```python
from build123d import *

# Parameters (mm, degrees)
BASPROSKE_W        = 13
BASPROSKE_H        = 16
TOOTHCUT_DEPTH     = 27.095976701
TEETHCUTS_COUNT    = 14
TEETHCUTS_ANGLE    = 334.285714286
BORSKE_R           = 4
BORE_DEPTH         = 50.0005588
SKETCH2_R          = 0.75
CUT_EXTRUDE1_DEPTH = 6
CIRPATTERN1_COUNT  = 4


with BuildPart() as part:
    # BasProSke → Base-Revolve (revolve)
    with BuildSketch(Plane(origin=(0, 0, 0), x_dir=(1, 0, 0), z_dir=(0, 1, 0)), mode=Mode.PRIVATE) as base_revolve_sk:
        with Locations((6.5, 8)):
            Rectangle(BASPROSKE_W, BASPROSKE_H)
    revolve(base_revolve_sk.sketch.rotate(Axis((-10, 0, 0), (1, 0, 0)), 180), axis=Axis((-10, 0, 0), (1, 0, 0)))

    # TooCutSke → ToothCut (cut, through all)
    with BuildSketch(Plane(origin=(0, 0, 0), x_dir=(0, 0, -1), z_dir=(1, 0, 0))):
        with BuildLine():
            ThreePointArc((1.067858192, 11.449309144), (0, 11.499), (-1.067858192, 11.449309144))
            ThreePointArc((-1.067858192, 11.449309144), (-1.641684211, 13.812780716), (-3.163375005, 15.710076503))
            ThreePointArc((-3.163375005, 15.710076503), (0, 16.0254), (3.163375005, 15.710076503))
            ThreePointArc((3.163375005, 15.710076503), (1.641684211, 13.812780716), (1.067858192, 11.449309144))
        make_face()
    toothcut = extrude(amount=TOOTHCUT_DEPTH, mode=Mode.SUBTRACT)

    # TeethCuts: ToothCut ×14 about axis
    teethcuts_axis = Axis((-10, 0, 0), (1, 0, 0))
    for i in range(1, TEETHCUTS_COUNT):
        add(toothcut.rotate(teethcuts_axis, i * TEETHCUTS_ANGLE / (TEETHCUTS_COUNT - 1)), mode=Mode.SUBTRACT)

    # BorSke → Bore (cut, symmetric)
    with BuildSketch(Plane(origin=(0, 0, 0), x_dir=(0, 0, -1), z_dir=(1, 0, 0))):
        with Locations(Location((0, 0, 0), (0, 0, 180))):
            Circle(BORSKE_R)
    extrude(amount=BORE_DEPTH, both=True, mode=Mode.SUBTRACT)

    # Sketch2 → Cut-Extrude1 (cut)
    with BuildSketch(Plane(origin=(13, 0, 0), x_dir=(0, 0, -1), z_dir=(1, 0, 0))):
        with Locations((-3.5, 7)):
            Circle(SKETCH2_R)
        with Locations((0, 7)):
            Circle(SKETCH2_R)
        with Locations((3.5, 7)):
            Circle(SKETCH2_R)
    cut_extrude1 = extrude(amount=-CUT_EXTRUDE1_DEPTH, mode=Mode.SUBTRACT)

    # CirPattern1: Cut-Extrude1 ×4 about axis
    cirpattern1_axis = Axis((0, 0, 0), (1, 0, 0))
    for i in range(1, CIRPATTERN1_COUNT):
        add(cut_extrude1.rotate(cirpattern1_axis, i * 360 / CIRPATTERN1_COUNT), mode=Mode.SUBTRACT)


solid = part.part
```
Here's how the part is built. I have some questions about the finished solid (model axes, mm). A direction names the side the tool comes from. Round coordinates to 2 decimals unless told otherwise and drop trailing zeros. Order: outer loops, then holes, each group sorted by start corner. A loop starts at its lowest first (then second) coordinate and runs counter-clockwise, first axis right, second up. Notation, with made-up numbers: (73.25, -37) -> (110.25, -37) arc R12 ccw to (110.25, -20) -> close; hole circle Ø1 at (-8.75, 9). An arc over 180 degrees is marked (long way). Use a Markdown table: item, result. Add a question column.
(1) I need wall thicknesses on line 1 along Y through (x, z) = (9.55, -7); line 2 along Z through (x, y) = (7.75, -10); line 3 along Z through (x, y) = (2, -7). Which ranges of each line are inside material? Lowest first, please.
(2) Suppose I cut it at C-C, the plane x = 9.5. Count the separate pieces of the cut face and the enclosed holes in it, and give its area (3 significant figures).
(3) Suppose I cut it at A-A, the plane z = 0. Please give me the cut outline in (x, y), and give its area (3 significant figures).
(4) For faces 4 (the face through (6.409, 10.367, 4.976)), 5 (the face through (10.042, -4.095, 6.544)), 6 (the face through (6.41, -13.77, -1.62)), which set-ups out of +Z, -Z, +X, -X, +Y, -Y let a thin tool reach every point of the face, with its end or its side?
(5) Suppose I cut it at D-D, the plane z = 7. Please give me the cut outline in (x, y).
(6) For pin 1 Ø4 at (x, y) = (11, -9.5) entering from +Z; pin 2 Ø5 at (x, z) = (11, -11) entering from -Y; pin 3 Ø4 at (x, y) = (6, 4.5) entering from +Z; pin 4 Ø5 at (y, z) = (0, 0) entering from -X, each with a flat end and sliding along its axis, tell me the tip position at first contact or that it passes through.
(7) Suppose I cut it at B-B, the plane z = -9. Please give me the cut outline in (x, y), and give its area (3 significant figures).
(8) If we mould it in two halves opening along Z, with no side actions, what happens to faces 1 (the face through (7, 0, -16)), 2 (the face through (6.591, 3.905, -0.867)), 3 (the face through (13, 3, -3))? For each: released by +Z, released by -Z, zero draft, split by the parting line, or undercut.
Verdict:
| question | item | result |
|---|---|---|
| 1 | line 1 | -11.32 to -4.25, -2.75 to -0.75, 0.75 to 2.75, 4.25 to 11.32 |
| 1 | line 2 | -9.82 to -6.01, -5.68 to 5.68, 6.01 to 9.82 |
| 1 | line 3 | -14.39 to -10.8, -9.12 to 9.12, 10.8 to 14.39 |
| 2 | separate pieces | 1 |
| 2 | enclosed holes | 13 |
| 2 | area | 512 mm2 |
| 3 | outline | (0, -11.5) -> (13, -11.5) -> (13, -7.75) -> (7, -7.75) -> (7, -6.25) -> (13, -6.25) -> (13, -4) -> (0, -4) -> close; (0, 4) -> (13, 4) -> (13, 6.25) -> (7, 6.25) -> (7, 7.75) -> (13, 7.75) -> (13, 11.5) -> (0, 11.5) -> close |
| 3 | area | 177 mm2 |
| 4 | face 4 | +X, -X |
| 4 | face 5 | +X |
| 4 | face 6 | +X, -X, -Y |
| 5 | outline | (0, -11.32) -> (13, -11.32) -> (13, -4.25) -> (7, -4.25) -> (7, -2.75) -> (13, -2.75) -> (13, -0.75) -> (7, -0.75) -> (7, 0.75) -> (13, 0.75) -> (13, 2.75) -> (7, 2.75) -> (7, 4.25) -> (13, 4.25) -> (13, 11.32) -> (0, 11.32) -> close |
| 6 | pin 1 | z = 10.26 |
| 6 | pin 2 | y = -12.77 |
| 6 | pin 3 | z = 14.57 |
| 6 | pin 4 | through |
| 7 | outline | (0, -12.58) -> (13, -12.58) -> (13, -8.68) -> (0, -8.68) -> close; (0, -7.16) -> (13, -7.16) -> (13, 7.16) -> (0, 7.16) -> close; (0, 8.68) -> (13, 8.68) -> (13, 12.58) -> (0, 12.58) -> close |
| 7 | area | 287 mm2 |
| 8 | face 1 | released by -Z |
| 8 | face 2 | undercut |
| 8 | face 3 | zero draft |
